Design review of the part shown in the three views and the two pictorial views. Dimensions are in mm from the part's minimum x, y and z. Round coordinates to 2 decimals unless told otherwise and drop trailing zeros. Loops run counter-clockwise (first coordinate to the right, second up) from the corner with the lowest first, then second, coordinate; pieces in that order, holes last. Notation, with made-up numbers: M -1.75,25 L 10.25,25 A19 cw 10.25,47 Z; hole C 79,67.5 d1. An arc over 180 degrees is marked long. Return JSON: item names as keys, results as strings. Group by question number.
Q1. Consider section C-C (x = 15). State the section outline as (y, z) points (1 decimal).
Q2. To check wall thickness, follow line 1 along X through (y, z) = (62.5, 123); line 2 along Z through (x, y) = (12.5, 41); line 3 along Z through (x, y) = (14.5, 43) (1 decimal). State the ranges of each line that lie inside material, in increasing order.
Q3. Consider section D-D (y = 46.5). State the section outline as (x, z) points, and give its area (3 significant figures).
Q4. Consider section B-B (z = 80.5). State the section outline as (x, y) points, and give its area (3 significant figures).
Q5. Clearance check with flat-ended pins moving along their axes: pin 1 Ø5 at (x, y) = (2.5, 32) entering from -Z; pin 2 Ø4 at (x, z) = (10, 28.5) entering from -Y; pin 3 Ø4 at (x, z) = (14.5, 79.5) entering from +Y. State where each tip first meets the part, or that it passes through.
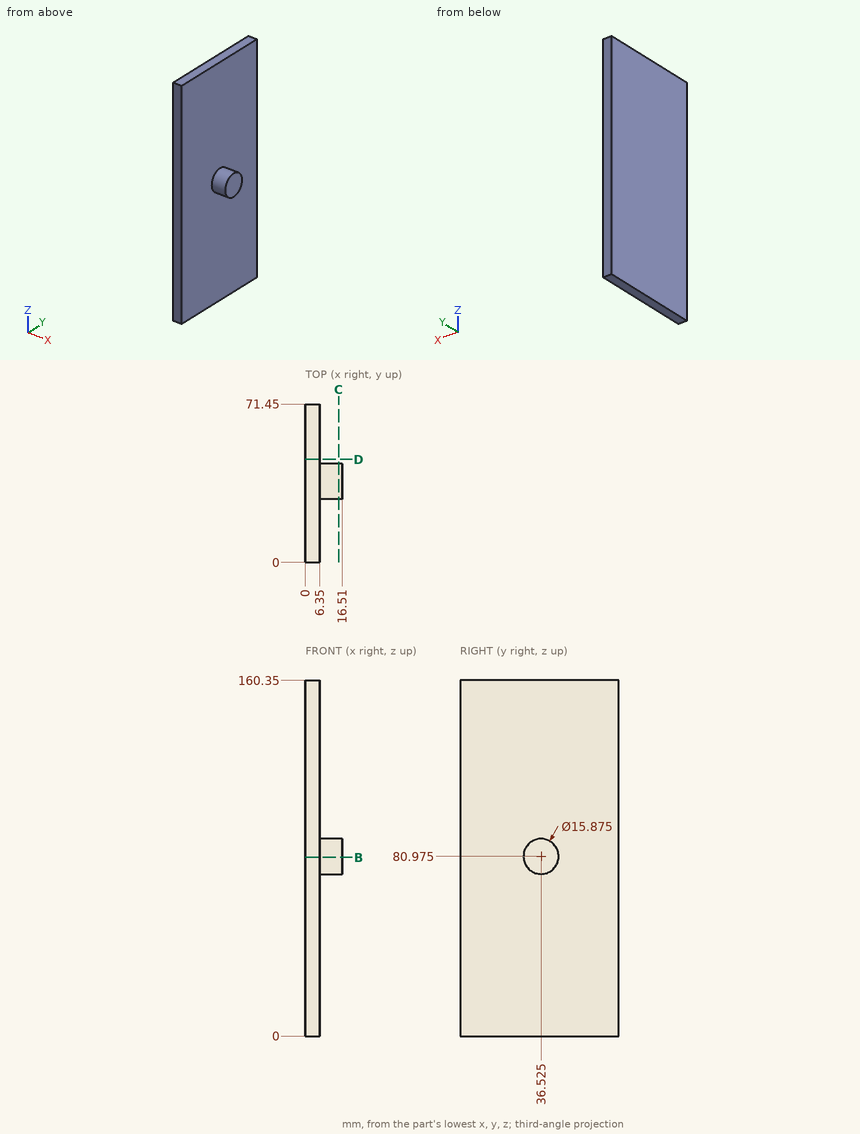
Values:
{
 "1": {"outline": "C 36.5,81 d15.9"},
 "2": {"line 1": "x = 0 to 6.35", "line 2": "z = 74.42 to 87.53", "line 3": "z = 76.4 to 85.6"},
 "3": {"outline": "M 0,0 L 6.35,0 L 6.35,160.35 L 0,160.35 Z", "area": "1,020 mm2"},
 "4": {"outline": "M 0,0 L 6.35,0 L 6.35,28.6 L 16.51,28.6 L 16.51,44.45 L 6.35,44.45 L 6.35,71.45 L 0,71.45 Z", "area": "615 mm2"},
 "5": {"pin 1": "stops at z = 0", "pin 2": "passes through", "pin 3": "stops at y = 44.46"}
}
